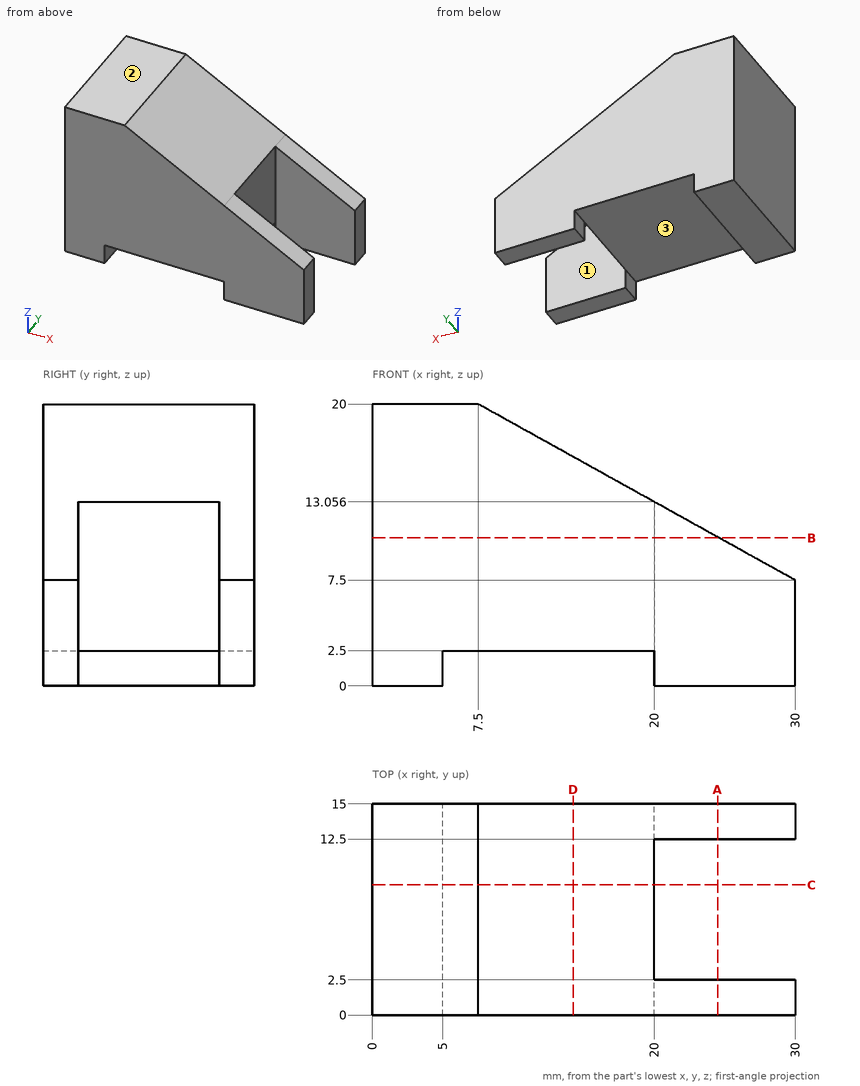
Check sheet for the drawn part. Datum: minimum x, y, z corner. Units: mm. A direction names the side the tool comes from. Round coordinates to 2 decimals unless told otherwise and drop trailing zeros. Loops run counter-clockwise (first coordinate to the right, second up) from the corner with the lowest first, then second, coordinate; pieces in that order, holes last. Notation, with made-up numbers: (84.5, 75) - (130.5, 75) arc R13 cw to (130.5, 79) - close; hole circle Ø10 at (55, 76). An arc over 180 degrees is marked (long way). Write item = value, one per line. Start each with the question number.
1. Section check C-C on y = 9.25. Enter the section's corners in (x, z) (1 decimal), then the cut area to 3 significant figures.
2. Thickness scan on line 1 (Y direction, x = 22.75, z = 2.25); line 2 (X direction, y = 8.75, z = 12.5); line 3 (Z direction, x = 16.5, y = 13.25). Record the ranges inside material, lowest first.
3. Set-up check for the marked faces 1, 2 and 3: record each of +Z, -Z, +X, -X, +Y, -Y from which the full face is reachable in a straight line by a thin tool's end or side.
4. Section check B-B on z = 10.5. Enter the section's corners in (x, y), then the cut area to 3 significant figures.
5. Section check D-D on x = 14.25. Enter the section's corners in (y, z), then the cut area to 3 significant figures.
6. Section check A-A on x = 24.5. Enter the section's corners in (y, z) (1 decimal).
7. Depth check by flat-ended pin: pin 1 (4 mm diameter, centred on x = 19, z = 17, fed in from +Y); pin 2 (3 mm diameter, centred on y = 12, z = 16.5, fed in from -X); pin 3 (1.2 mm diameter, centred on y = 5, z = 1.5, fed in from +X); pin 4 (1 mm diameter, centred on x = 19, y = 12.5, fed in from +Z). Enter the tip coordinate at first touch or a pass-through.
Working result:
q1.outline = (0, 0) - (5, 0) - (5, 2.5) - (20, 2.5) - (20, 13.1) - (7.5, 20) - (0, 20) - close
q1.area = 319 mm^2
q2.line_1 = 0 to 2.5, 12.5 to 15
q2.line_2 = 0 to 20
q2.line_3 = 2.5 to 15
q3.face_1 = +Z, -Z, +X
q3.face_2 = +Z, +X, -X, +Y, -Y
q3.face_3 = -Z, +Y, -Y
q4.outline = (0, 0) - (24.6, 0) - (24.6, 2.5) - (20, 2.5) - (20, 12.5) - (24.6, 12.5) - (24.6, 15) - (0, 15) - close
q4.area = 323 mm^2
q5.outline = (0, 2.5) - (15, 2.5) - (15, 16.25) - (0, 16.25) - close
q5.area = 206 mm^2
q6.outline = (0, 0) - (2.5, 0) - (2.5, 10.6) - (0, 10.6) - close; (12.5, 0) - (15, 0) - (15, 10.6) - (12.5, 10.6) - close
q7.pin_1 = through
q7.pin_2 = 0
q7.pin_3 = 5
q7.pin_4 = 13.89
